```python
from build123d import *

# Parameters (mm, degrees)
SKETCH1_W           = 14.097
SKETCH1_H           = 14.097
BOSS_EXTRUDE1_DEPTH = 10.541
SKETCH2_R           = 3.81
BOSS_EXTRUDE2_DEPTH = 5.08
BOSS_EXTRUDE3_DEPTH = 4.826
SKETCH4_W           = 22.86
SKETCH4_H           = 22.86
BOSS_EXTRUDE4_DEPTH = 1.143
SKETCH5_W           = 22.86
SKETCH5_H           = 15.24
BOSS_EXTRUDE5_DEPTH = 27.051


with BuildPart() as part:
    # Sketch1 → Boss-Extrude1 (new body)
    with BuildSketch(Plane.XY):
        Rectangle(SKETCH1_W, SKETCH1_H)
    extrude(amount=BOSS_EXTRUDE1_DEPTH)

    # Sketch2 → Boss-Extrude2 (add)
    with BuildSketch(Plane.XY.offset(10.541)):
        Circle(SKETCH2_R)
    extrude(amount=BOSS_EXTRUDE2_DEPTH)

    # Sketch3 → Boss-Extrude3 (add)
    with BuildSketch(Plane(origin=(0, 0, 0), x_dir=(-1, 0, 0), z_dir=(0, 0, -1))):
        with BuildLine():
            Line((-9.525, 2.032), (-7.0485, 2.032))
            Line((-7.0485, 2.032), (-7.0485, -2.032))
            Line((-7.0485, -2.032), (-9.525, -2.032))
            ThreePointArc((-9.525, -2.032), (-11.557, 0), (-9.525, 2.032))
        make_face()
    boss_extrude3 = extrude(amount=-BOSS_EXTRUDE3_DEPTH)

    # Mirror1: Boss-Extrude3 across plane
    add(boss_extrude3.mirror(Plane(origin=(0, 0, 0), x_dir=(0, 0, 1), z_dir=(1, 0, 0))))

    # Sketch4 → Boss-Extrude4 (add)
    with BuildSketch(Plane(origin=(0, 0, 0), x_dir=(-1, 0, 0), z_dir=(0, 0, -1))):
        Rectangle(SKETCH4_W, SKETCH4_H)
    extrude(amount=BOSS_EXTRUDE4_DEPTH)

    # Sketch5 → Boss-Extrude5 (add)
    with BuildSketch(Plane(origin=(0, 0, -1.143), x_dir=(-1, 0, 0), z_dir=(0, 0, -1))):
        Rectangle(SKETCH5_W, SKETCH5_H)
    extrude(amount=BOSS_EXTRUDE5_DEPTH)


solid = part.part
```
The model under review builds one solid part; all positions refer to its coordinate system, in mm. A direction names the side the tool comes from. Round coordinates to 2 decimals unless told otherwise and drop trailing zeros. Loops run counter-clockwise (first coordinate to the right, second up) from the corner with the lowest first, then second, coordinate; pieces in that order, holes last. Notation, with made-up numbers: (46.25, -30.75) -> (74.25, -30.75) arc R20 ccw to (74.25, -13.75) -> close; hole circle Ø8 at (79.25, 49.5). An arc over 180 degrees is marked (long way). Answer in a Markdown table with one row per item.
1) Tool access review of faces 1 (the flat face through (0, -9, -1.143)), 2 (the flat face through (-11.43, 0, -14)), 3 (the flat face through (0, 7.62, -14)), 4 (the flat face through (9, 0, 4.826)), 5 (the flat face through (-3, -3, 10.541)): name each direction out of +Z, -Z, +X, -X, +Y, -Y from which nothing blocks a thin tool from reaching the whole face with its end or side.
Taken from the geometry:
| item | result |
|---|---|
| face 1 | -Z, +X, -X, -Y |
| face 2 | -Z, -X, +Y, -Y |
| face 3 | -Z, +X, -X, +Y |
| face 4 | +Z, +X, +Y, -Y |
| face 5 | +Z |
2) Consider section B-B, the plane y = 0. Write out the cut boundary in (x, z), plus the area to 3 significant figures.
Taken from the geometry:
| item | result |
|---|---|
| outline | (-11.56, 0) -> (-11.43, 0) -> (-11.43, -28.19) -> (11.43, -28.19) -> (11.43, 0) -> (11.56, 0) -> (11.56, 4.83) -> (7.05, 4.83) -> (7.05, 10.54) -> (3.81, 10.54) -> (3.81, 15.62) -> (-3.81, 15.62) -> (-3.81, 10.54) -> (-7.05, 10.54) -> (-7.05, 4.83) -> (-11.56, 4.83) -> close |
| area | 875 mm² |
3) Wall thickness on line 1 along X through (y, z) = (1.5, -0.5); line 2 along Z through (x, y) = (5.5, -8); line 3 along X through (y, z) = (-2.5, 6.5): over which ranges is each line inside the solid? List them lowest first.
Taken from the geometry:
| item | result |
|---|---|
| line 1 | x = -11.43 to 11.43 |
| line 2 | z = -1.14 to 0 |
| line 3 | x = -7.05 to 7.05 |
4) Consider section A-A, the plane z = 3. Write out the cut boundary in (x, y) (1 decimal), plus the area to 3 significant figures.
Taken from the geometry:
| item | result |
|---|---|
| outline | (-9.5, -2) -> (-7, -2) -> (-7, -7) -> (7, -7) -> (7, -2) -> (9.5, -2) arc R2 ccw to (9.5, 2) -> (7, 2) -> (7, 7) -> (-7, 7) -> (-7, 2) -> (-9.5, 2) arc R2 ccw to start |
| area | 232 mm² |
5) Consider section D-D, the plane y = -8.5. Write out the cut boundary in (x, z).
Taken from the geometry:
| item | result |
|---|---|
| outline | (-11.43, -1.14) -> (11.43, -1.14) -> (11.43, 0) -> (-11.43, 0) -> close |
6) Consider section C-C, the plane x = 0. Write out the cut boundary in (y, z).
Taken from the geometry:
| item | result |
|---|---|
| outline | (-11.43, -1.14) -> (-7.62, -1.14) -> (-7.62, -28.19) -> (7.62, -28.19) -> (7.62, -1.14) -> (11.43, -1.14) -> (11.43, 0) -> (7.05, 0) -> (7.05, 10.54) -> (3.81, 10.54) -> (3.81, 15.62) -> (-3.81, 15.62) -> (-3.81, 10.54) -> (-7.05, 10.54) -> (-7.05, 0) -> (-11.43, 0) -> close |
7) For pin 1 Ø3 at (x, z) = (-4.5, 2) entering from -Y; pin 2 Ø2.5 at (x, z) = (8, 3.5) entering from +Y; pin 3 Ø3 at (y, z) = (-5, -11.5) entering from +X, all flat-tipped, find the tip position at first contact; note any pin that passes through.
Taken from the geometry:
| item | result |
|---|---|
| pin 1 | stops at y = -7.05 |
| pin 2 | stops at y = 7.05 |
| pin 3 | stops at x = 11.43 |
